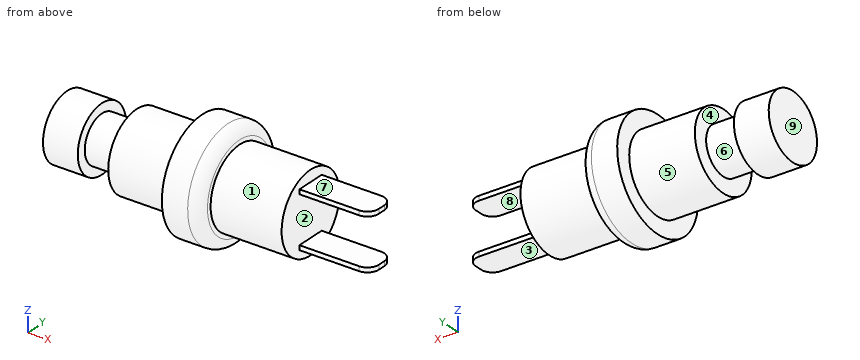
```python
from build123d import *

# Parameters (mm, degrees)
FILLET1_R           = 1
SKETCH2_W           = 0.4
SKETCH2_H           = 2.65
BOSS_EXTRUDE1_DEPTH = 6.22
FILLET2_R           = 1


with BuildPart() as part:
    # Sketch1 → Revolve1 (revolve)
    with BuildSketch(Plane.XY, mode=Mode.PRIVATE) as revolve1_sk:
        Polygon((25.103538705, 0), (3.767538705, 0), (3.767538705, 2.883), (6.815538705, 2.883), (6.815538705, 2.049985706), (9.863538705, 2.049985706), (9.863538705, 3.397), (15.616538705, 3.397), (15.616538705, 4.832), (18.880538705, 4.832), (18.880538705, 3.457874146), (25.103538705, 3.457874146), align=None)
    revolve(revolve1_sk.sketch.rotate(Axis((0, 0, 0), (1, 0, 0)), 90), axis=Axis((0, 0, 0), (1, 0, 0)))

    # Fillet1
    fillet1_edges = [part.edges().sort_by_distance(p)[0] for p in [
        (18.880538705, 0, -4.832),
    ]]
    fillet(fillet1_edges, radius=FILLET1_R)

    # Sketch2 → Boss-Extrude1 (add)
    with BuildSketch(Plane(origin=(25.103538705, 0, 0), x_dir=(0, 0, -1), z_dir=(1, 0, 0))):
        with Locations((-2.25, 0)):
            Rectangle(SKETCH2_W, SKETCH2_H)
        with Locations((2.25, 0)):
            Rectangle(SKETCH2_W, SKETCH2_H)
    extrude(amount=BOSS_EXTRUDE1_DEPTH)

    # Fillet2
    fillet2_edges = [part.edges().sort_by_distance(p)[0] for p in [
        (31.323538705, 1.325, 2.25),
        (31.323538705, -1.325, 2.25),
        (31.323538705, 1.325, -2.25),
        (31.323538705, -1.325, -2.25),
    ]]
    fillet(fillet2_edges, radius=FILLET2_R)


solid = part.part
```
Verification items for the finished model (mm, model axes). Face numbers are marked on the shaded views. A direction names the side the tool comes from. Coordinates: 2 decimals unless noted, no trailing zeros. Write each loop counter-clockwise with the first axis right and the second up, starting at its lowest first coordinate (ties: lowest second). Pieces come first, ordered by that corner, then holes. Notation, with made-up numbers: M -18,46 L 0,46 A13 cw 0,65 Z; hole C 47,-16.75 d1. An arc over 180 degrees is marked long. Answer as a JSON object with one key per item and string values. Group by question number.
(1) Gauge pin test, flat ends, axial feed: pin 1 (1.3 mm diameter, centred on x = 29, y = 0, fed in from -Z); pin 2 (4 mm diameter, centred on y = 3, z = -2, fed in from +X); pin 3 (1.3 mm diameter, centred on x = 28.5, y = -0.5, fed in from +Z). Record the tip position at first contact, or that the pin passes through.
(2) Cross-section at A-A, the plane x = 28.5. Record the cut outline in (y, z) (3 decimals), and give its area (3 significant figures).
(3) Material ranges on line 1 (X direction, y = 1.75, z = 0.5); line 2 (X direction, y = 1.5, z = -2.5); line 3 (X direction, y = 1.5, z = 2), recorded low to high.
(4) Tool access check on the marked faces 5, 6, 7, 8 and 9. Record the directions out of +Z, -Z, +X, -X, +Y, -Y that give a thin tool (end or side, any length) a straight path to the whole face; none if there is none.
(5) Cross-section at C-C, the plane x = 18.25. Record the cut outline in (y, z), and give its area (3 significant figures).
(6) Release check for a two-part mould opening along Z. For the marked faces 1, 2, 3 and 4 record: +Z half, -Z half, draft (parallel to the pull), parting line (faces both ways), or undercut.
(7) Cross-section at B-B, the plane z = 0. Record the cut outline in (x, y), and give its area (3 significant figures).
Reply:
{
 "1": {"pin 1": "z = -2.45", "pin 2": "x = 31.06", "pin 3": "z = 2.45"},
 "2": {"outline": "M -1.325,-2.45 L 1.325,-2.45 L 1.325,-2.05 L -1.325,-2.05 Z; M -1.325,2.05 L 1.325,2.05 L 1.325,2.45 L -1.325,2.45 Z", "area": "2.12 mm²"},
 "3": {"line 1": "3.77 to 25.1", "line 2": "9.86 to 25.1", "line 3": "3.77 to 6.82, 9.86 to 25.1"},
 "4": {"face 5": "-X", "face 6": "none", "face 7": "+Z, +X, +Y, -Y", "face 8": "+X, +Y, -Y", "face 9": "+Z, -Z, -X, +Y, -Y"},
 "5": {"outline": "C 0,0 d9.52", "area": "71.2 mm²"},
 "6": {"face 1": "parting line", "face 2": "undercut", "face 3": "-Z half", "face 4": "draft"},
 "7": {"outline": "M 3.77,-2.88 L 6.82,-2.88 L 6.82,-2.05 L 9.86,-2.05 L 9.86,-3.4 L 15.62,-3.4 L 15.62,-4.83 L 17.88,-4.83 A1 ccw 18.88,-3.83 L 18.88,-3.46 L 25.1,-3.46 L 25.1,3.46 L 18.88,3.46 L 18.88,3.83 A1 ccw 17.88,4.83 L 15.62,4.83 L 15.62,3.4 L 9.86,3.4 L 9.86,2.05 L 6.82,2.05 L 6.82,2.88 L 3.77,2.88 Z", "area": "143 mm²"}
}
